Can you work these out from the drawing? Everything is in mm from the part's minimum corner. A direction names the side the tool comes from. Coordinates: 2 decimals unless noted, no trailing zeros. Order: outer loops, then holes, each group sorted by start corner. A loop starts at its lowest first (then second) coordinate and runs counter-clockwise, first axis right, second up. Notation, with made-up numbers: (78, -35) -> (82, -35) arc R22 cw to (82, -1) -> close; hole circle Ø6 at (1.25, 41.5). An arc over 180 degrees is marked (long way). Use a Markdown table: item, result. Add a question column.
1) If we section it at A-A (y = 28): Write out the boundary of the cut face in (x, z), plus the area to 3 significant figures.
2) If we section it at C-C (x = 15): Write out the boundary of the cut face in (y, z).
3) Will these pins go through, and if not, where does the flat tip stop? pin 1 Ø3 at (y, z) = (42.5, 269.5) entering from +X; pin 2 Ø18.5 at (x, y) = (55.5, 15) entering from +Z; pin 3 Ø6 at (x, z) = (52.5, 67.5) entering from -Y; pin 4 Ø1 at (y, z) = (36.5, 128.5) entering from -X.
4) Thinking about a two-plate mould opening in X: for the marked faces 3, 4 and 5, which applies, +X half, -X half, draft (parallel to the pull), parting line (faces both ways), or undercut?
5) If we section it at B-B (z = 119): Write out the boundary of the cut face in (x, y).
6) If we section it at D-D (x = 34.5): Write out the boundary of the cut face in (y, z).
7) Which directions (+Z, -Z, +X, -X, +Y, -Y) give clear straight access to the entire face, cutting with the end or side of a thin tool? Please do the marked faces 1 and 2.
8) If I drill on L1, parallel to X at y = 2, z = 189; L2, parallel to Y at x = 15.5, z = 75; L3, parallel to Z at x = 58, y = 5, over which ranges is the centre line in solid material (lowest first)? Write a range as [from, to].
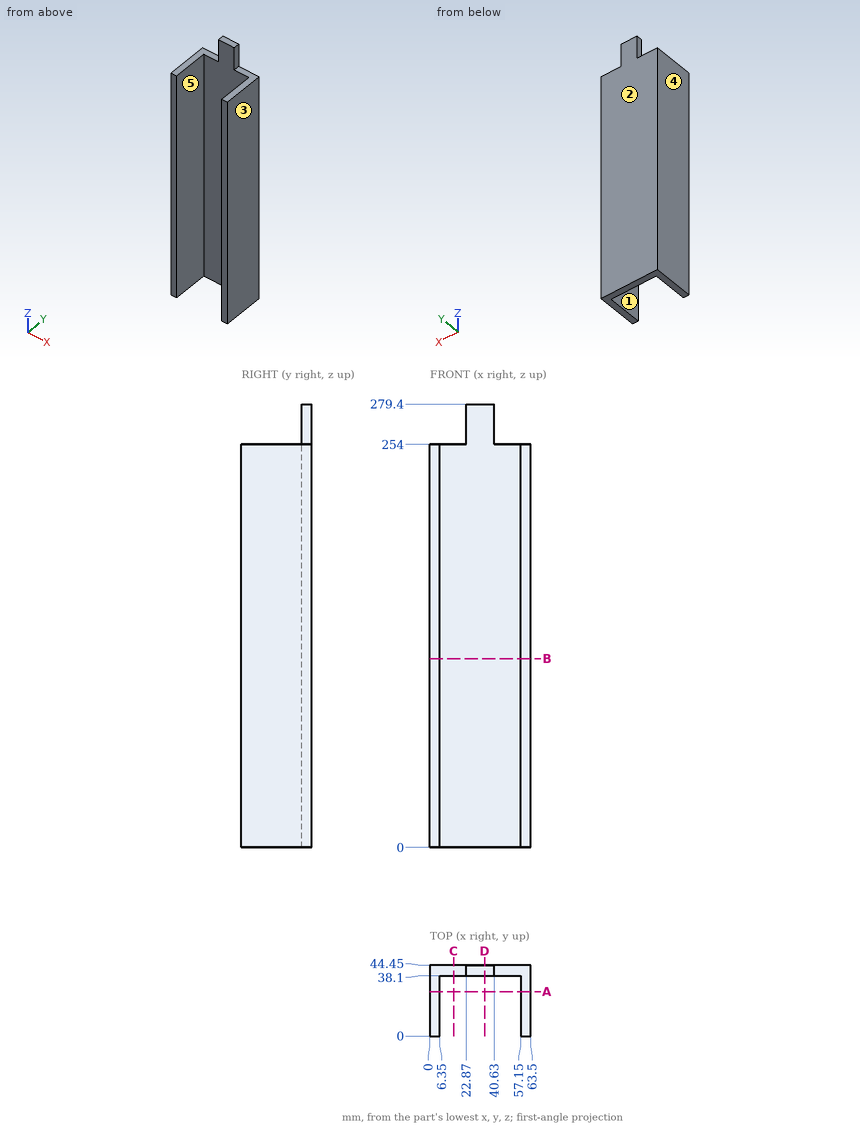
Answer sheet:
| question | item | result |
|---|---|---|
| 1 | outline | (0, 0) -> (6.35, 0) -> (6.35, 254) -> (0, 254) -> close; (57.15, 0) -> (63.5, 0) -> (63.5, 254) -> (57.15, 254) -> close |
| 1 | area | 3,230 mm2 |
| 2 | outline | (38.1, 0) -> (44.45, 0) -> (44.45, 254) -> (38.1, 254) -> close |
| 3 | pin 1 | x = 40.63 |
| 3 | pin 2 | z = 254 |
| 3 | pin 3 | y = 38.1 |
| 3 | pin 4 | x = 0 |
| 4 | face 3 | +X half |
| 4 | face 4 | -X half |
| 4 | face 5 | undercut |
| 5 | outline | (0, 0) -> (6.35, 0) -> (6.35, 38.1) -> (57.15, 38.1) -> (57.15, 0) -> (63.5, 0) -> (63.5, 44.45) -> (0, 44.45) -> close |
| 6 | outline | (38.1, 0) -> (44.45, 0) -> (44.45, 279.4) -> (38.1, 279.4) -> close |
| 7 | face 1 | +Z, -Z, -Y |
| 7 | face 2 | +Z, -Z, +X, -X, +Y |
| 8 | L1 | [0, 6.35], [57.15, 63.5] |
| 8 | L2 | [38.1, 44.45] |
| 8 | L3 | [0, 254] |
